For this review, take the finished solid that the model builds, in its own axes (mm). A direction names the side the tool comes from. Give positions to 0.01 mm unless a question says otherwise; leave off trailing zeros. Loops run counter-clockwise (first coordinate to the right, second up) from the corner with the lowest first, then second, coordinate; pieces in that order, holes last. Notation, with made-up numbers: (4.5, 71.5) - (33.5, 71.5) arc R21 cw to (33.5, 109.5) - close; hole circle Ø3 at (68.5, 65.5). An arc over 180 degrees is marked (long way). Use CSV: the item, a comma, the result in double quotes. Start each with the question number.
1. Take a section at A-A on x = -17. Give the boundary of the cut face in (y, z), plus the area to 3 significant figures.
2. Take a section at C-C on y = 0.55. Give the boundary of the cut face in (x, z).
3. Take a section at B-B on z = -46. Give the boundary of the cut face in (x, y), plus the area to 3 significant figures.
4. Take a section at D-D on z = -5. Give the boundary of the cut face in (x, y), plus the area to 3 significant figures.
5. Wall thickness on line 1 (X direction, y = 1.55, z = -5); line 2 (Z direction, x = -9.5, y = 0.4); line 3 (Z direction, x = -51, y = 1.25): over which ranges is each line inside the solid? List them lowest first.
6. Mouldability with a two-part tool opening along X and no side actions: class faces 5 (the flat face through (-50, 1, -36)), 6 (the flat face through (-19, 1, 4)), 7 (the flat face through (-16, 1, -16.5)) as pulls with the +X half, pulls with the -X half, needs draft (parallel to the pull), parting line crosses it, or undercut.
7. For pin 1 (1 mm diameter, centred on y = 1.5, z = -21.5, fed in from -X); pin 2 (1 mm diameter, centred on y = 1, z = 2.5, fed in from -X); pin 3 (1 mm diameter, centred on x = -31.5, y = 1.5, fed in from +Z), all flat-tipped, find the tip position at first contact; note any pin that passes through.
8. For faces 1 (the flat face through (-18.5, 1, -22)), 2 (the flat face through (-10, 1, 0)), 3 (the flat face through (-34, 1, -52)), 4 (the flat face through (-14, 1, -52)), list the 3-axis set-ups (+Z, -Z, +X, -X, +Y, -Y) from which the entire face can be reached by the end or side of a thin tool; tool diameter is ignored.
Autodesk Inventor part; units mm, degrees
ref_plane "YZ Plane" through (0, 0, 0) normal (1, 0, 0) x (0, 1, 0)
ref_plane "XZ Plane" through (0, 0, 0) normal (0, 1, 0) x (-1, 0, 0)
ref_plane "XY Plane" through (0, 0, 0) normal (0, 0, 1) x (1, 0, 0)
sketch "Boceto1" plane through (0, 0, 0) normal (0, 1, 0) x (-1, 0, 0)
  line L0 (48, 0) -> (48, -51)
  line L1 (48, -51) -> (0, -51)
  line L2 (0, -51) -> (0, 0)
  line L3 (24, 7.5) -> (29, 7.5)
  line L4 (29, 7.5) -> (29, 0)
  line L5 (24, 7.5) -> (19, 7.5)
  line L6 (19, 7.5) -> (19, 0)
  line L7 (24, 7.5) -> (24, -1.25)
  circle A0 centre (24, -1.25) radius 1.5
  line L8 (29, 0) -> (48, 0)
  line L9 (19, 0) -> (0, 0)
  dimension "d0" = 48
  dimension "d1" = 51
  dimension "d3" = 5
  dimension "d4" = 5
  dimension "d5" = 8.75
  dimension "d6" = 3
extrude "Extrusión1" add sketch "Boceto1" along normal blind 2
ref_plane "Plano de trabajo1" through (-48, -25, -47.5) normal (0, -1, 0) x (1, 0, 0)
sketch "Boceto4" plane through (0, 2, 0) normal (0, 1, 0) x (1, 0, 0)
  line L0 (0, 51) -> (-48, 51)
  line L1 (-24, 51) -> (-24, 53)
  line L2 (-24, 53) -> (-34, 53)
  line L3 (-34, 53) -> (-34, 51)
  line L4 (-34, 51) -> (-14, 51)
  line L5 (-14, 51) -> (-14, 53)
  line L6 (-14, 53) -> (-24, 53)
  point P0 (0, 0)
  dimension "d18" = 2
  dimension "d19" = 10
  dimension "d20" = 20
extrude "Extrusión4" add sketch "Boceto4" against normal blind 2
sketch "Boceto6" plane through (0, 2, 0) normal (0, 1, 0) x (1, 0, 0)
  line L0 (-48, 47.5) -> (-48, 31.5)
  line L1 (-48, 47.5) -> (-18.5, 47.5)
  line L2 (-18.5, 47.5) -> (-18.5, 26.5)
  line L3 (-18.5, 26.5) -> (-18.5, 16.5)
  line L4 (-18.5, 16.5) -> (-12.5, 16.5)
  line L5 (-12.5, 16.5) -> (-12.5, 26.5)
  line L6 (-12.5, 26.5) -> (-18.5, 26.5)
  point P0 (0, 0)
  dimension "d26" = 29.5
  dimension "d27" = 21
  dimension "d28" = 10
  dimension "d29" = 6
extrude "Extrusión6" cut sketch "Boceto6" against normal blind 2
sketch "Boceto7" plane through (0, 2, 0) normal (0, 1, 0) x (1, 0, 0)
  circle A0 centre (-24, 1.25) radius 1.5
  circle A1 centre (-24, 1.25) radius 1.5
  point P0 (0, 0)
extrude "Extrusión7" add sketch "Boceto7" against normal blind 2
sketch "Boceto8" plane through (0, 2, 0) normal (0, 1, 0) x (1, 0, 0)
  line L0 (-48, 51) -> (-48, 0)
  line L1 (-48, 51) -> (-48, 31.5)
  line L2 (-48, 31.5) -> (-50, 31.5)
  line L3 (-50, 31.5) -> (-50, 41)
  line L4 (-50, 41) -> (-54, 41)
  line L5 (-54, 41) -> (-54, 51)
  line L6 (-54, 51) -> (-48, 51)
  point P0 (0, 0)
  dimension "d34" = 19.5
  dimension "d35" = 2
  dimension "d36" = 9.5
  dimension "d37" = 4
extrude "Extrusión8" add sketch "Boceto8" against normal blind 2
sketch "Boceto9" plane through (0, 2, 0) normal (0, 1, 0) x (1, 0, 0)
  line L0 (-48, 0) -> (-29, 0)
  line L1 (-48, 0) -> (-48, 5)
  line L2 (-48, 31.5) -> (-48, 0)
  line L3 (-48, 5) -> (-38.5, 5)
  line L4 (-48, 5) -> (-9.5, 5)
  circle A0 centre (-38.5, 5) radius 1.5
  circle A1 centre (-9.5, 5) radius 1.5
  line L5 (0, 51) -> (-14, 51)
  line L6 (0, 51) -> (0, 41)
  line L7 (0, 0) -> (0, 51)
  line L8 (0, 41) -> (-3.75, 41)
  circle A2 centre (-3.75, 41) radius 1.5
  line L9 (-34, 51) -> (-54, 51)
  line L10 (-54, 51) -> (-51, 51)
  line L11 (-51, 51) -> (-51, 46)
  circle A3 centre (-51, 46) radius 1.5
  dimension "d40" = 5
  dimension "d41" = 9.5
  dimension "d42" = 38.5
  dimension "d43" = 3
  dimension "d44" = 3
  dimension "d45" = 10
  dimension "d46" = 3.75
  dimension "d47" = 3
  dimension "d48" = 3
  dimension "d49" = 3
extrude "Extrusión9" cut sketch "Boceto9" against normal blind 2
properties part number "arm_2_case"
Check result:
1,outline,"(0, -53) - (2, -53) - (2, -26.5) - (0, -26.5) - close; (0, -16.5) - (2, -16.5) - (2, 0) - (0, 0) - close"
1,area,"86.0 mm²"
2,outline,"(-54, -51) - (-34, -51) - (-34, -53) - (-14, -53) - (-14, -51) - (0, -51) - (0, 0) - (-19, 0) - (-19, 7.5) - (-29, 7.5) - (-29, 0) - (-48, 0) - (-48, -31.5) - (-50, -31.5) - (-50, -41) - (-54, -41) - close; hole circle Ø3 at (-51, -46); hole circle Ø3 at (-38.5, -5); hole (-18.5, -26.5) - (-12.5, -26.5) - (-12.5, -16.5) - (-18.5, -16.5) - close; hole circle Ø3 at (-9.5, -5); hole circle Ø3 at (-3.75, -41)"
3,outline,"(-54, 0) - (-52.5, 0) - (-52.5, 2) - (-54, 2) - close; (-49.5, 0) - (0, 0) - (0, 2) - (-49.5, 2) - close"
3,area,"102 mm²"
4,outline,"(-48, 0) - (-40, 0) - (-40, 2) - (-48, 2) - close; (-37, 0) - (-11, 0) - (-11, 2) - (-37, 2) - close; (-8, 0) - (0, 0) - (0, 2) - (-8, 2) - close"
4,area,"84.0 mm²"
5,line 1,"x = -48 to -40, -37 to -11, -8 to 0"
5,line 2,"z = -51 to -6.5, -3.5 to 0"
5,line 3,"z = -51 to -47.5, -44.5 to -41"
6,face 5,"pulls with the -X half"
6,face 6,"pulls with the +X half"
6,face 7,"undercut"
7,pin 1,"stops at x = -48"
7,pin 2,"stops at x = -29"
7,pin 3,"stops at z = 0"
8,face 1,"+Y, -Y"
8,face 2,"+Z, +X, +Y, -Y"
8,face 3,"-Z, -X, +Y, -Y"
8,face 4,"-Z, +X, +Y, -Y"
